Print and shaded views of the part. All mm, measured from the part's lowest x, y and z. Coordinates: 2 decimals unless noted, no trailing zeros. Loops run counter-clockwise (first coordinate to the right, second up) from the corner with the lowest first, then second, coordinate; pieces in that order, holes last. Notation, with made-up numbers: M 30,86.25 L 42,86.25 A18 cw 42,103.25 Z; hole C -16,21.25 d2. An arc over 180 degrees is marked long. Use a Markdown table: item, result. Add a question column.
1) Band-saw the part on D-D (z = 3.5). List the corners of the cut face in (x, y).
2) Pin check, flat tips, straight feed: pin 1 Ø3 at (x, z) = (11, 18.5) entering from -Y; pin 2 Ø6 at (y, z) = (29.5, 12) entering from +X (1 decimal); pin 3 Ø5 at (x, z) = (28, 19) entering from +Y. Stop position of each tip, or through.
3) Wall check: probe 1 along Y at (x, z) = (22, 20.9); probe 2 along Y at (x, z) = (21.5, 1.5) (1 decimal); probe 3 along X at (y, z) = (37, 14) (1 decimal). Give the ranges that are in metal, low to high. Write a range as from..to.
4) Pull direction Y, two halves, no side cores. Call the marked faces 1, 2 and 3: released by +Y, released by -Y, zero draft, split by the parting line, or undercut.
5) Band-saw the part on C-C (x = 26.5). List the corners of the cut face in (y, z) (1 decimal).
6) Band-saw the part on B-B (y = 24.5). List the corners of the cut face in (x, z).
7) Band-saw the part on A-A (x = 22). List the corners of the cut face in (y, z).
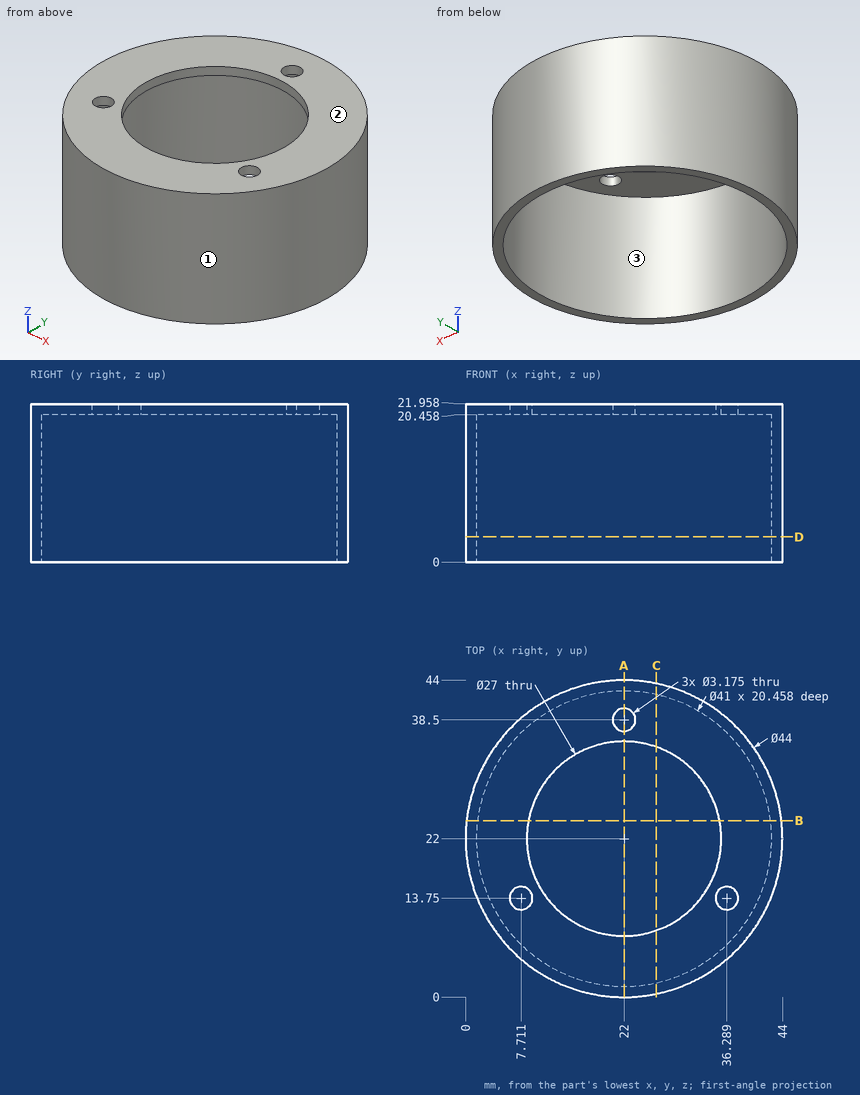
Entries:
| question | item | result |
|---|---|---|
| 1 | outline | C 22,22 d44; hole C 22,22 d41 |
| 2 | pin 1 | y = 2.16 |
| 2 | pin 2 | x = 43.5 |
| 2 | pin 3 | y = 43.72 |
| 3 | probe 1 | 0..8.5, 35.5..36.91, 40.09..44 |
| 3 | probe 2 | 0..1.5, 42.5..44 |
| 3 | probe 3 | 5.9..8, 36..38.1 |
| 4 | face 1 | split by the parting line |
| 4 | face 2 | zero draft |
| 4 | face 3 | undercut |
| 5 | outline | M 0.5,0 L 2,0 L 2,20.5 L 9.3,20.5 L 9.3,22 L 0.5,22 Z; M 34.7,20.5 L 42,20.5 L 42,0 L 43.5,0 L 43.5,22 L 34.7,22 Z |
| 6 | outline | M 0.14,0 L 1.65,0 L 1.65,20.46 L 8.73,20.46 L 8.73,21.96 L 0.14,21.96 Z; M 35.27,20.46 L 42.35,20.46 L 42.35,0 L 43.86,0 L 43.86,21.96 L 35.27,21.96 Z |
| 7 | outline | M 0,0 L 1.5,0 L 1.5,20.46 L 8.5,20.46 L 8.5,21.96 L 0,21.96 Z; M 35.5,20.46 L 36.91,20.46 L 36.91,21.96 L 35.5,21.96 Z; M 40.09,20.46 L 42.5,20.46 L 42.5,0 L 44,0 L 44,21.96 L 40.09,21.96 Z |
